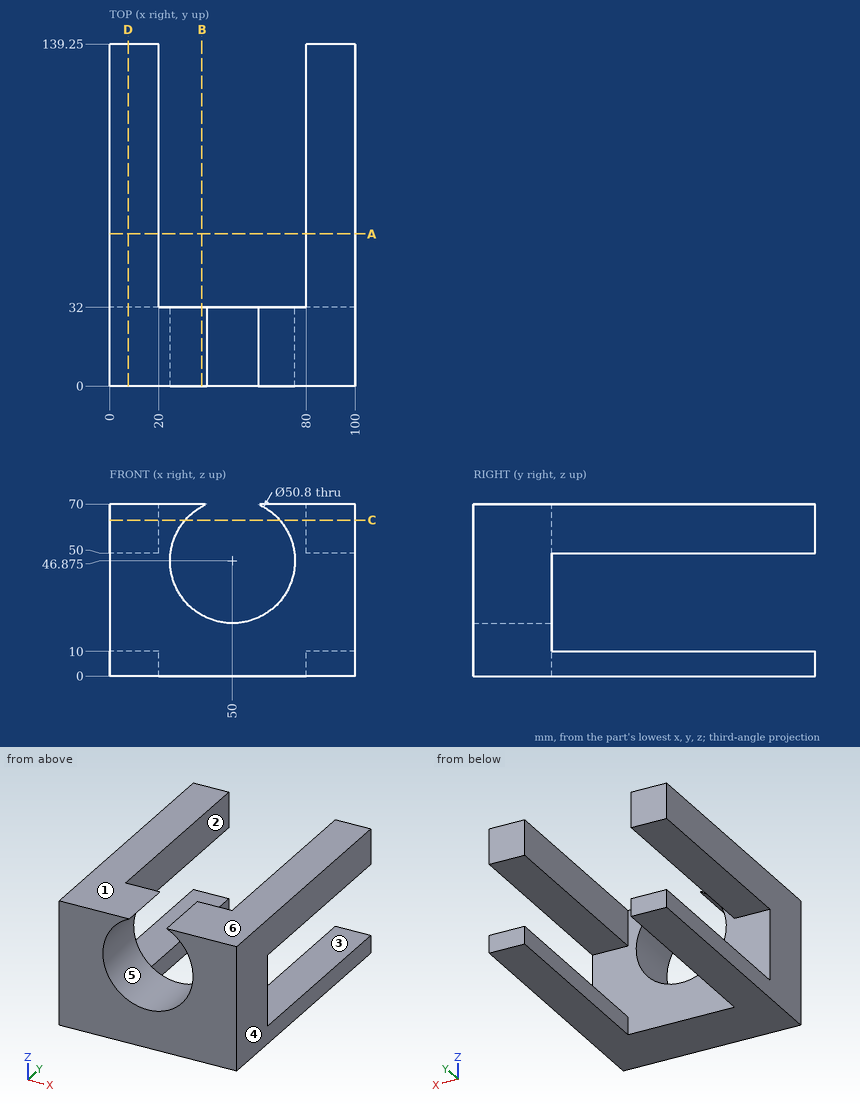
Source: three-view drawing plus pictorial views. Frame: mm from the lowest corner of the part. A direction names the side the tool comes from. Coordinates: 2 decimals unless noted, no trailing zeros. Order: outer loops, then holes, each group sorted by start corner. A loop starts at its lowest first (then second) coordinate and runs counter-clockwise, first axis right, second up. Notation, with made-up numbers: M 55.25,59.25 L 64.25,59.25 A29 cw 64.25,94.25 Z; hole C -16,-18 d9. An arc over 180 degrees is marked long. Answer in a Markdown table with one row per item.
(1) Section query D-D, the plane x = 7.5. Output: boundary loops of the cut face in (y, z), plus the area to 3 significant figures.
Numbers:
| item | result |
|---|---|
| outline | M 0,0 L 139.25,0 L 139.25,10 L 32,10 L 32,50 L 139.25,50 L 139.25,70 L 0,70 Z |
| area | 5,460 mm^2 |
(2) Section query A-A, the plane y = 62. Output: boundary loops of the cut face in (x, z).
Numbers:
| item | result |
|---|---|
| outline | M 0,0 L 20,0 L 20,10 L 0,10 Z; M 0,50 L 20,50 L 20,70 L 0,70 Z; M 80,0 L 100,0 L 100,10 L 80,10 Z; M 80,50 L 100,50 L 100,70 L 80,70 Z |
(3) Access query for the marked faces 1, 2 and 3. Directions: +Z, -Z, +X, -X, +Y, -Y. A direction counts if a zero-diameter tool reaches every point of the face in a straight line with its end or side. Return the directions, or none.
Numbers:
| item | result |
|---|---|
| face 1 | +Z, +X, -X, +Y, -Y |
| face 2 | +Z, -Z, +Y |
| face 3 | +X, -X, +Y |
(4) Draft query along Z for the marked faces 4, 5 and 6. Return one class per face: pulls with the +Z half, pulls with the -Z half, needs draft (parallel to the pull), parting line crosses it, or undercut.
Numbers:
| item | result |
|---|---|
| face 4 | needs draft |
| face 5 | undercut |
| face 6 | pulls with the +Z half |
(5) Contact query for flat-ended pins moving along their axis: pin 1 Ø4 at (x, z) = (71, 59) entering from +Y; pin 2 Ø5 at (x, y) = (44.5, 15.5) entering from +Z; pin 3 Ø4 at (y, z) = (122.5, 13.5) entering from +X. Output: stop coordinate, or through.
Numbers:
| item | result |
|---|---|
| pin 1 | stops at y = 32 |
| pin 2 | stops at z = 22.77 |
| pin 3 | passes through |
(6) Material intervals for line 1 (X direction, y = 107, z = 62.5); line 2 (Z direction, x = 7, y = 70); line 3 (Z direction, x = 50, y = 11) (3 decimals), sorted ascending. Write a range as [from, to].
Numbers:
| item | result |
|---|---|
| line 1 | x = [0, 20], [80, 100] |
| line 2 | z = [0, 10], [50, 70] |
| line 3 | z = [0, 21.475] |
(7) Section query C-C, the plane z = 63.5. Output: boundary loops of the cut face in (x, y), plus the area to 3 significant figures.
Numbers:
| item | result |
|---|---|
| outline | M 0,0 L 30.8,0 L 30.8,32 L 20,32 L 20,139.25 L 0,139.25 Z; M 69.2,0 L 100,0 L 100,139.25 L 80,139.25 L 80,32 L 69.2,32 Z |
| area | 6,260 mm^2 |
(8) Section query B-B, the plane x = 37.5. Output: boundary loops of the cut face in (y, z).
Numbers:
| item | result |
|---|---|
| outline | M 0,0 L 32,0 L 32,24.76 L 0,24.76 Z; M 0,68.99 L 32,68.99 L 32,70 L 0,70 Z |
